Verification items for this drawing (mm, ordinates from the low corner). A direction names the side the tool comes from. Coordinates: 2 decimals unless noted, no trailing zeros. Write each loop counter-clockwise with the first axis right and the second up, starting at its lowest first coordinate (ties: lowest second). Pieces come first, ordered by that corner, then holes. Notation, with made-up numbers: M 65,15.25 L 80,15.25 A29 cw 80,52.25 Z; hole C 40,11.5 d11. An arc over 180 degrees is marked long. Write each question's results on one line, items separated by ' | '.
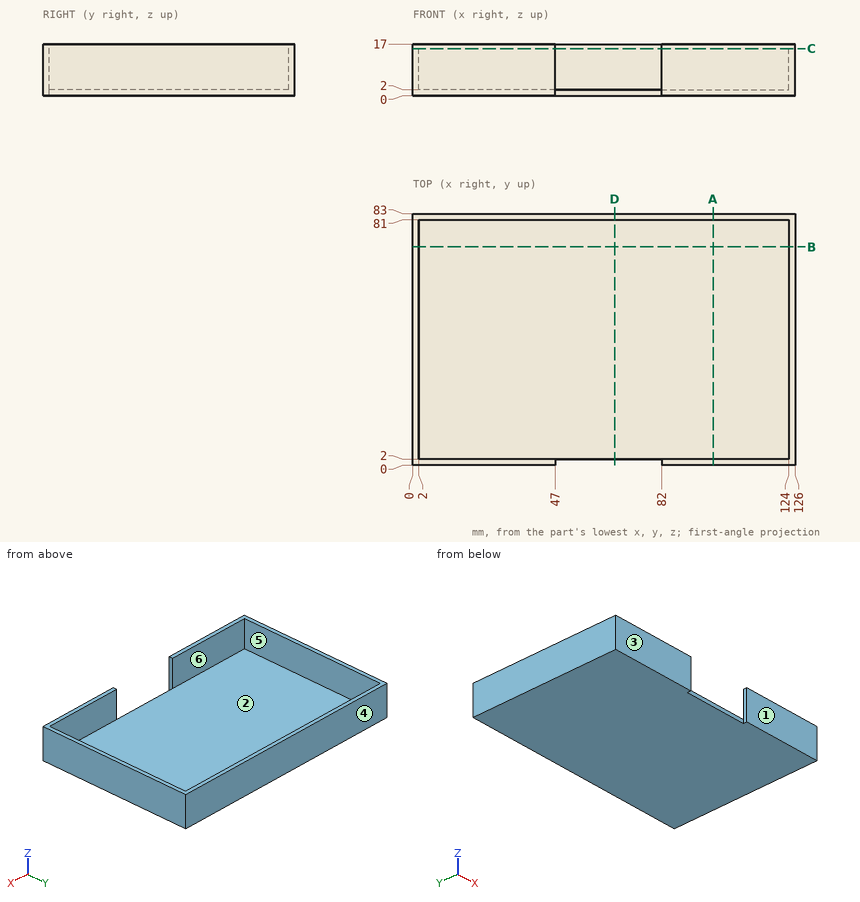
Q1. Sectioned sample at A-A on x = 99. Record the cut outline in (y, z), and give its area (3 significant figures).
Geometry check:
outline: M 0,0 L 83,0 L 83,17 L 81,17 L 81,2 L 2,2 L 2,17 L 0,17 Z | area: 226 mm2
Q2. Depth check by flat-ended pin: P1, Ø6, axis at x = 40.5, y = 22, coming from the +Z side; P2, Ø0.6, axis at x = 67, z = 0.5, coming from the -Y side; P3, Ø8, axis at x = 98, y = 43, coming from the -Z side; P4, Ø3, axis at x = 64.5, z = 9.5, coming from the -Y side. Enter the tip coordinate at first touch or a pass-through.
Geometry check:
P1: stops at z = 2 | P2: stops at y = 2 | P3: stops at z = 0 | P4: stops at y = 81
Q3. Sectioned sample at C-C on z = 15.5. Record the cut outline in (x, y), and give its area (3 significant figures).
Geometry check:
outline: M 0,0 L 47,0 L 47,2 L 2,2 L 2,81 L 124,81 L 124,2 L 82,2 L 82,0 L 126,0 L 126,83 L 0,83 Z | area: 750 mm2
Q4. Sectioned sample at D-D on x = 66.5. Record the cut outline in (y, z).
Geometry check:
outline: M 2,0 L 83,0 L 83,17 L 81,17 L 81,2 L 2,2 Z
Q5. Scan lines: probe 1 along Y at (x, z) = (108.5, 14.75); probe 2 along X at (y, z) = (16.5, 3); probe 3 along Z at (x, y) = (34, 64). Record each from-to range of solid material in increasing order.
Geometry check:
probe 1: y = 0 to 2, 81 to 83 | probe 2: x = 0 to 2, 124 to 126 | probe 3: z = 0 to 2
Q6. Mould release check, pull along Y, two halves, no side actions. Record for the marked faces 3, 4, 5 and 6: pulls with the +Y half, pulls with the -Y half, needs draft (parallel to the pull), parting line crosses it, or undercut.
Geometry check:
face 3: pulls with the -Y half | face 4: pulls with the +Y half | face 5: undercut | face 6: undercut
Q7. Access from +Z, -Z, +X, -X, +Y, -Y to the whole of each face (thin tool, end or side, straight path). Record for the marked faces 1 and 2.
Geometry check:
face 1: +Z, -Z, +X, -X, -Y | face 2: +Z
Q8. Sectioned sample at B-B on y = 72. Record the cut outline in (x, z), and give its area (3 significant figures).
Geometry check:
outline: M 0,0 L 126,0 L 126,17 L 124,17 L 124,2 L 2,2 L 2,17 L 0,17 Z | area: 312 mm2
